from build123d import *

# Parameters (mm, degrees)
F0_W     = 79.375
F0_H     = 15.875
F0_R     = 2.38125
F1_DEPTH = 3.175
F2_DEPTH = 4.7625
F3_T     = -1.5875
F4_R     = 3.175
F4_R_2   = 2.38125
F5_DEPTH = 1.5875


with BuildPart() as f1:
    # F0 (on Top) → F1 (new body)
    with BuildSketch(Plane.XY):
        with Locations((23.8125, -3.96875)):
            Rectangle(F0_W, F0_H)
        with Locations((-11.90625, -7.9375)):
            Circle(F0_R, mode=Mode.SUBTRACT)
        with Locations((-3.96875, -7.9375)):
            Circle(F0_R, mode=Mode.SUBTRACT)
        with Locations((3.96875, -7.9375)):
            Circle(F0_R, mode=Mode.SUBTRACT)
        with Locations((11.90625, -7.9375)):
            Circle(F0_R, mode=Mode.SUBTRACT)
        with Locations((19.84375, -7.9375)):
            Circle(F0_R, mode=Mode.SUBTRACT)
        with Locations((27.78125, -7.9375)):
            Circle(F0_R, mode=Mode.SUBTRACT)
        with Locations((35.71875, -7.9375)):
            Circle(F0_R, mode=Mode.SUBTRACT)
        with Locations((43.65625, -7.9375)):
            Circle(F0_R, mode=Mode.SUBTRACT)
        with Locations((51.59375, -7.9375)):
            Circle(F0_R, mode=Mode.SUBTRACT)
        with Locations((59.53125, -7.9375)):
            Circle(F0_R, mode=Mode.SUBTRACT)
        with Locations((-11.90625, 0)):
            Circle(F0_R, mode=Mode.SUBTRACT)
        with Locations((-3.96875, 0)):
            Circle(F0_R, mode=Mode.SUBTRACT)
        with Locations((3.96875, 0)):
            Circle(F0_R, mode=Mode.SUBTRACT)
        with Locations((11.90625, 0)):
            Circle(F0_R, mode=Mode.SUBTRACT)
        with Locations((19.84375, 0)):
            Circle(F0_R, mode=Mode.SUBTRACT)
        with Locations((27.78125, 0)):
            Circle(F0_R, mode=Mode.SUBTRACT)
        with Locations((35.71875, 0)):
            Circle(F0_R, mode=Mode.SUBTRACT)
        with Locations((43.65625, 0)):
            Circle(F0_R, mode=Mode.SUBTRACT)
        with Locations((51.59375, 0)):
            Circle(F0_R, mode=Mode.SUBTRACT)
        with Locations((59.53125, 0)):
            Circle(F0_R, mode=Mode.SUBTRACT)
    extrude(amount=F1_DEPTH)

    # F0 (on Top) → F2 (join)
    with BuildSketch(Plane.XY):
        with Locations((-11.90625, 0)):
            Circle(F0_R)
        with Locations((-11.90625, -7.9375)):
            Circle(F0_R)
        with Locations((-3.96875, -7.9375)):
            Circle(F0_R)
        with Locations((-3.96875, 0)):
            Circle(F0_R)
        with Locations((3.96875, 0)):
            Circle(F0_R)
        with Locations((3.96875, -7.9375)):
            Circle(F0_R)
        with Locations((11.90625, -7.9375)):
            Circle(F0_R)
        with Locations((11.90625, 0)):
            Circle(F0_R)
        with Locations((19.84375, 0)):
            Circle(F0_R)
        with Locations((27.78125, 0)):
            Circle(F0_R)
        with Locations((27.78125, -7.9375)):
            Circle(F0_R)
        with Locations((19.84375, -7.9375)):
            Circle(F0_R)
        with Locations((35.71875, 0)):
            Circle(F0_R)
        with Locations((43.65625, 0)):
            Circle(F0_R)
        with Locations((43.65625, -7.9375)):
            Circle(F0_R)
        with Locations((35.71875, -7.9375)):
            Circle(F0_R)
        with Locations((51.59375, 0)):
            Circle(F0_R)
        with Locations((59.53125, 0)):
            Circle(F0_R)
        with Locations((59.53125, -7.9375)):
            Circle(F0_R)
        with Locations((51.59375, -7.9375)):
            Circle(F0_R)
    extrude(amount=F2_DEPTH)

    # F3
    f3_openings = [f1.faces().sort_by_distance(p)[0] for p in [
        (23.8125, -3.96875, 0),
    ]]
    offset(amount=F3_T, openings=f3_openings, kind=Kind.INTERSECTION)

    # F4 (on face) → F5 (join)
    with BuildSketch(Plane(origin=(0, 0, 1.5875), x_dir=(1, 0, 0), z_dir=(0, 0, -1))):
        with BuildLine():
            ThreePointArc((-4.7625, 3.96875), (-6.7224801022, 6.9020675157), (-10.1825640303, 6.2138140303))
            Line((-10.1825640303, 6.2138140303), (-9.6212980227, 5.6525480227))
            ThreePointArc((-9.6212980227, 5.6525480227), (-7.0262350767, 6.1687381368), (-5.55625, 3.96875))
            ThreePointArc((-5.55625, 3.96875), (-5.7375118632, 3.0574850767), (-6.2537019773, 2.2849519773))
            Line((-6.2537019773, 2.2849519773), (-5.6924359697, 1.7236859697))
            ThreePointArc((-5.6924359697, 1.7236859697), (-5.0041824843, 2.7537301022), (-4.7625, 3.96875))
        make_face()
        with BuildLine():
            Line((-9.6212980227, 5.6525480227), (-10.1825640303, 6.2138140303))
            ThreePointArc((-10.1825640303, 6.2138140303), (-10.1825640303, 1.7236859697), (-5.6924359697, 1.7236859697))
            Line((-5.6924359697, 1.7236859697), (-6.2537019773, 2.2849519773))
            ThreePointArc((-6.2537019773, 2.2849519773), (-9.6212980227, 2.2849519773), (-9.6212980227, 5.6525480227))
        make_face()
        with Locations((0, 3.96875)):
            Circle(F4_R)
        with Locations((0, 3.96875)):
            Circle(F4_R_2, mode=Mode.SUBTRACT)
        with Locations((7.9375, 3.96875)):
            Circle(F4_R)
        with Locations((7.9375, 3.96875)):
            Circle(F4_R_2, mode=Mode.SUBTRACT)
        with Locations((15.875, 3.96875)):
            Circle(F4_R)
        with Locations((15.875, 3.96875)):
            Circle(F4_R_2, mode=Mode.SUBTRACT)
        with Locations((23.8125, 3.96875)):
            Circle(F4_R)
        with Locations((23.8125, 3.96875)):
            Circle(F4_R_2, mode=Mode.SUBTRACT)
        with Locations((31.75, 3.96875)):
            Circle(F4_R)
        with Locations((31.75, 3.96875)):
            Circle(F4_R_2, mode=Mode.SUBTRACT)
        with Locations((39.6875, 3.96875)):
            Circle(F4_R)
        with Locations((39.6875, 3.96875)):
            Circle(F4_R_2, mode=Mode.SUBTRACT)
        with Locations((47.625, 3.96875)):
            Circle(F4_R)
        with Locations((47.625, 3.96875)):
            Circle(F4_R_2, mode=Mode.SUBTRACT)
        with Locations((55.5625, 3.96875)):
            Circle(F4_R)
        with Locations((55.5625, 3.96875)):
            Circle(F4_R_2, mode=Mode.SUBTRACT)
    extrude(amount=F5_DEPTH)


solid = f1.part
Design review of the part built by this model. Coordinates are the model's own, in mm. A direction names the side the tool comes from. Round coordinates to 2 decimals unless told otherwise and drop trailing zeros. Write each loop counter-clockwise with the first axis right and the second up, starting at its lowest first coordinate (ties: lowest second). Pieces come first, ordered by that corner, then holes. Notation, with made-up numbers: (88.5, 74.25) - (92.5, 74.25) arc R26 cw to (92.5, 98.25) - close; hole circle Ø8 at (-29.5, -28). An arc over 180 degrees is marked (long way). Use a Markdown table: item, result. Add a question column.
1. We need section C-C (x = 32.5). State the section outline as (y, z) points (1 decimal).
2. We need section A-A (z = 0.65). Count the separate pieces of the cut face and the enclosed holes in it, then the cut area to 3 significant figures.
3. Mouldability with a two-part tool opening along Y and no side actions: class faces 1 (the face through (-4, 0, 4.762)), 2 (the face through (23, -4, 3.175)), 3 (the face through (-12, 0, 3.175)) as +Y half, -Y half, draft (parallel to the pull), parting line (faces both ways), or undercut.
4. Wall thickness on probe 1 along Y at (x, z) = (0, 0.9); probe 2 along Y at (x, z) = (35.5, 3.5); probe 3 along Y at (x, z) = (34.5, 1.55): over which ranges is each line inside the solid? List them lowest first.
5. Clearance check with flat-ended pins moving along their axes: pin 1 (1.3 mm diameter, centred on x = 59.5, y = 0, fed in from -Z) (3 decimals); pin 2 (1 mm diameter, centred on x = 28, y = -2.5, fed in from -Z); pin 3 (6 mm diameter, centred on x = 18.5, y = -8.5, fed in from -Z). State where each tip first meets the part, or that it passes through.
6. For faces 4 (the face through (18.146, -4.684, 0.805)), 5 (the face through (25.9, -9.4, 4)), list the 3-axis set-ups (+Z, -Z, +X, -X, +Y, -Y) from which the entire face can be reached by the end or side of a thin tool; tool diameter is ignored.
Output:
| question | item | result |
|---|---|---|
| 1 | outline | (-11.9, 0) - (-10.3, 0) - (-10.3, 1.6) - (-7.1, 1.6) - (-7.1, 0) - (-6.2, 0) - (-6.2, 1.6) - (-1.7, 1.6) - (-1.7, 0) - (-0.9, 0) - (-0.9, 1.6) - (2.4, 1.6) - (2.4, 0) - (4, 0) - (4, 3.2) - (-11.9, 3.2) - close |
| 2 | separate pieces | 10 |
| 2 | enclosed holes | 10 |
| 2 | area | 417 mm2 |
| 3 | face 1 | draft |
| 3 | face 2 | undercut |
| 3 | face 3 | undercut |
| 4 | probe 1 | y = -11.91 to -10.32, -7.14 to -6.35, -1.59 to -0.79, 2.38 to 3.97 |
| 4 | probe 2 | y = -10.31 to -5.57, -2.37 to 2.37 |
| 4 | probe 3 | y = -11.91 to -10.32, -5.56 to -2.38, 2.38 to 3.97 |
| 5 | pin 1 | stops at z = 3.175 |
| 5 | pin 2 | stops at z = 1.59 |
| 5 | pin 3 | stops at z = 0 |
| 6 | face 4 | -Z |
| 6 | face 5 | +Z |
